Geometry check sheet. Reference: the model listing, model coordinates, mm. Face numbers are marked on the shaded views. A direction names the side the tool comes from. Give positions to 0.01 mm unless a question says otherwise; leave off trailing zeros. Order: outer loops, then holes, each group sorted by start corner. A loop starts at its lowest first (then second) coordinate and runs counter-clockwise, first axis right, second up. Notation, with made-up numbers: (69.25, 32) - (117.25, 32) arc R16 ccw to (117.25, 45) - close; hole circle Ø4 at (45.5, 59). An arc over 180 degrees is marked (long way). Put each result on its own line as item: value. Start each with the question number.
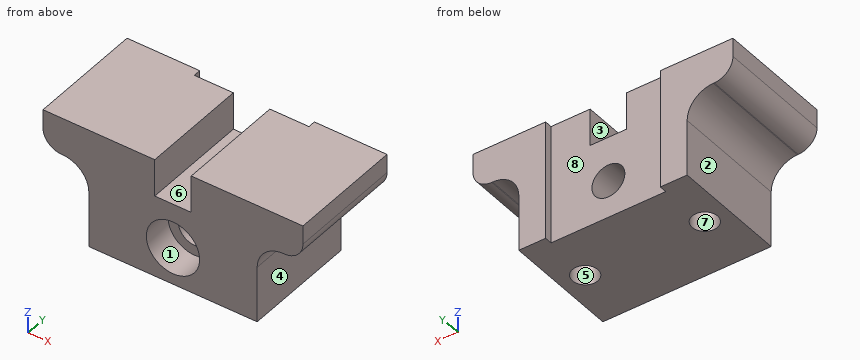
```python
from build123d import *

# Parameters (mm, degrees)
F1_DEPTH       = 31
F3_DEPTH       = 2
F5_D           = 6.8
F5_DEPTH       = 20
F5_TIP         = 2.0429261047
F7_D           = 8.8
F7_CBORE_D     = 14.25
F7_CBORE_DEPTH = 8


with BuildPart() as f1:
    # F0 (on Front) → F1 (new body)
    with BuildSketch(Plane.XZ):
        with BuildLine():
            Line((-4.875, 32), (-34.75, 32))
            Line((-34.75, 32), (-34.75, 27))
            ThreePointArc((-34.75, 27), (-33.2855339059, 23.4644660941), (-29.75, 22))
            Line((-29.75, 22), (-29.5, 22))
            ThreePointArc((-29.5, 22), (-24.5502525317, 19.9497474683), (-22.5, 15))
            Line((-22.5, 15), (-22.5, 0))
            Line((-22.5, 0), (22.5, 0))
            Line((22.5, 0), (22.5, 15))
            ThreePointArc((22.5, 15), (24.5502525317, 19.9497474683), (29.5, 22))
            Line((29.5, 22), (29.75, 22))
            ThreePointArc((29.75, 22), (33.2855339059, 23.4644660941), (34.75, 27))
            Line((34.75, 27), (34.75, 32))
            Line((34.75, 32), (4.875, 32))
            Line((4.875, 32), (4.875, 22))
            Line((4.875, 22), (-4.875, 22))
            Line((-4.875, 22), (-4.875, 32))
        make_face()
    extrude(amount=F1_DEPTH)

    # F2 (on face) → F3 (cut)
    with BuildSketch(Plane(origin=(0, 0, 0), x_dir=(-1, 0, 0), z_dir=(0, 1, 0))):
        Polygon((15.325, 0), (15.325, 32), (4.875, 32), (4.875, 22), (-4.875, 22), (-4.875, 32), (-15.325, 32), (-15.325, 0), align=None)
    extrude(amount=-F3_DEPTH, mode=Mode.SUBTRACT)

    # F5
    with Locations(Plane(origin=(0, 0, 0), x_dir=(1, 0, 0), z_dir=(0, 0, -1))):
        with Locations((-16, 15.5), (16, 15.5)):
            Hole(F5_D / 2, depth=F5_DEPTH)
            with Locations((0, 0, -(F5_DEPTH + F5_TIP / 2))):  # 118° drill point
                Cone(0, F5_D / 2, F5_TIP, mode=Mode.SUBTRACT)

    # F7 (through all)
    with Locations(Plane.XZ.offset(31)):
        with Locations((0, 10)):
            CounterBoreHole(F7_D / 2, F7_CBORE_D / 2, F7_CBORE_DEPTH)


solid = f1.part
```
Item 1: Thickness scan on line 1 along Z through (x, y) = (0, -27) (3 decimals); line 2 along X through (y, z) = (-0.5, 10) (3 decimals); line 3 along Y through (x, z) = (16, 9.75). Record the ranges inside material, lowest first.
Item 2: Cross-section at B-B (x = 0). Enter the section's corners in (y, z) (3 decimals).
Item 3: Cross-section at C-C (y = -7.5). Enter the section's corners in (x, z) (3 decimals), and give its area (3 significant figures).
Item 4: Cross-section at A-A (z = 29). Enter the section's corners in (x, y) (3 decimals), and give its area (3 significant figures).
Item 5: Set-up check for the marked faces 1, 2, 3 and 4: record each of +Z, -Z, +X, -X, +Y, -Y from which the full face is reachable in a straight line by a thin tool's end or side.
Item 6: Release check for a two-part mould opening along Y. For the marked faces 5, 6, 7 and 8 record: +Y half, -Y half, draft (parallel to the pull), parting line (faces both ways), or undercut.
Item 7: Cross-section at D-D (z = 12). Enter the section's corners in (x, y) (3 decimals).
Item 8: Gauge pin test, flat ends, axial feed: pin 1 Ø3 at (x, y) = (-2, -24.5) entering from +Z; pin 2 Ø1 at (x, z) = (6, 6.5) entering from +Y; pin 3 Ø4 at (y, z) = (-6.5, 17.5) entering from +X. Record the tip position at first contact, or that the pin passes through.
Recorded:
1. line 1: z = 0 to 2.875, 17.125 to 22
1. line 2: x = -22.5 to -15.325, 15.325 to 22.5
1. line 3: y = -31 to -18.9, -12.1 to 0
2. outline: (-31, 0) - (-2, 0) - (-2, 5.6) - (-23, 5.6) - (-23, 2.875) - (-31, 2.875) - close; (-31, 17.125) - (-23, 17.125) - (-23, 14.4) - (-2, 14.4) - (-2, 22) - (-31, 22) - close
3. outline: (-34.75, 27) arc R5 ccw to (-29.75, 22) - (-29.5, 22) arc R7 cw to (-22.5, 15) - (-22.5, 0) - (22.5, 0) - (22.5, 15) arc R7 cw to (29.5, 22) - (29.75, 22) arc R5 ccw to (34.75, 27) - (34.75, 32) - (4.875, 32) - (4.875, 22) - (-4.875, 22) - (-4.875, 32) - (-34.75, 32) - close; hole circle Ø8.8 at (0, 10)
3. area: 1,540 mm^2
4. outline: (-34.75, -31) - (-4.875, -31) - (-4.875, -2) - (-15.325, -2) - (-15.325, 0) - (-34.75, 0) - close; (4.875, -31) - (34.75, -31) - (34.75, 0) - (15.325, 0) - (15.325, -2) - (4.875, -2) - close
4. area: 1,810 mm^2
5. face 1: -Y
5. face 2: -Z, -X, +Y, -Y
5. face 3: +Z, +Y, -Y
5. face 4: -Z, +X, +Y, -Y
6. face 5: undercut
6. face 6: draft
6. face 7: undercut
6. face 8: +Y half
7. outline: (-22.5, -31) - (-6.839, -31) - (-6.839, -23) - (-3.919, -23) - (-3.919, -2) - (-15.325, -2) - (-15.325, 0) - (-22.5, 0) - close; (3.919, -23) - (6.839, -23) - (6.839, -31) - (22.5, -31) - (22.5, 0) - (15.325, 0) - (15.325, -2) - (3.919, -2) - close; hole circle Ø6.8 at (-16, -15.5); hole circle Ø6.8 at (16, -15.5)
8. pin 1: stops at z = 22
8. pin 2: stops at y = -2
8. pin 3: stops at x = 24.14
